Input: part model. Units: mm. Frame: model coordinates. Coordinates: 2 decimals unless noted, no trailing zeros. Write item = value, one per line. Start each with the question number.
from build123d import *

# Parameters (mm, degrees)
SHELL1_T                = -1.2
SKETCH5_W               = 1.35
SKETCH5_H               = 5.256968873
SKETCH5_H_2             = 1.35
SKETCH5_W_2             = 5.491330354
SKETCH5_W_3             = 5.273072972
SKETCH5_H_3             = 5.618351113
BOSS_EXTRUDE1_DEPTH     = 4
SKETCH6_R               = 2.5
BOSS_EXTRUDE2_DEPTH     = 10
CUT_EXTRUDE3_DEPTH      = 10
CUT_EXTRUDE3_DEPTH_BACK = 10
CUT_EXTRUDE4_DEPTH      = 0.5


with BuildPart() as part:
    # Loft1: read off the stored shape, not the designer's step
    # Loft1: loft between two sections, ruled curve by curve
    loft1_from = [
        Edge.make_line((-10, 0, 9.05), (-10, 0, -9.05)),
        Edge.make_line((-10, 0, -9.05), (10, 0, -9.05)),
        Edge.make_line((10, 0, 9.05), (-10, 0, 9.05)),
        Edge.make_line((10, 0, -9.05), (10, 0, 9.05)),
    ]
    loft1_to = [
        Edge.make_line((-7.5, 10, 6.318777005), (-7.5, 10, -7.681222995)),
        Edge.make_line((-7.5, 10, -7.681222995), (7.5, 10, -7.681222995)),
        Edge.make_line((7.5, 10, 6.318777005), (-7.5, 10, 6.318777005)),
        Edge.make_line((7.5, 10, -7.681222995), (7.5, 10, 6.318777005)),
    ]
    loft1 = Solid(Shell([*[Face.make_surface_from_curves(loft1_from[k], loft1_to[k]) for k in range(4)], Face(Wire(loft1_from)), Face(Wire(loft1_to))]))
    add(loft1)

    # Shell1
    shell1_openings = [part.faces().sort_by_distance(p)[0] for p in [
        (0, 0, 0),
    ]]
    offset(amount=SHELL1_T, openings=shell1_openings, kind=Kind.INTERSECTION)

    # Sketch5 → Boss-Extrude1 (add)
    with BuildSketch(Plane(origin=(0, 10, 0), x_dir=(1, 0, 0), z_dir=(0, 1, 0))):
        with Locations((0, -2.44038684)):
            Rectangle(SKETCH5_W, SKETCH5_H)
        with Locations((0, 0.863097596)):
            Rectangle(SKETCH5_W, SKETCH5_H_2)
        with Locations((3.420665177, 0.863097596)):
            Rectangle(SKETCH5_W_2, SKETCH5_H_2)
        with Locations((-3.311536486, 0.863097596)):
            Rectangle(SKETCH5_W_3, SKETCH5_H_2)
        with Locations((0, 4.347273152)):
            Rectangle(SKETCH5_W, SKETCH5_H_3)
    extrude(amount=-BOSS_EXTRUDE1_DEPTH)

    # Sketch6 → Boss-Extrude2 (add)
    with BuildSketch(Plane(origin=(0, 10, 0), x_dir=(1, 0, 0), z_dir=(0, 1, 0))):
        with Locations(Location((0, 0.829201721, 0), (0, 0, 270))):
            Circle(SKETCH6_R)
        Polygon((-0.675, 2.913097596), (-0.675, 1.538097596), (-2.05, 1.538097596), (-2.05, 0.188097596), (-0.675, 0.188097596), (-0.675, -1.186902404), (0.675, -1.186902404), (0.675, 0.188097596), (2.05, 0.188097596), (2.05, 1.538097596), (0.675, 1.538097596), (0.675, 2.913097596), align=None, mode=Mode.SUBTRACT)
    extrude(amount=-BOSS_EXTRUDE2_DEPTH)

    # Sketch4 → Cut-Extrude3 (cut, two sides: drawn at the far end of the back side and taken through both)
    with BuildSketch(Plane.XY.offset(-CUT_EXTRUDE3_DEPTH_BACK)):
        with BuildLine():
            Line((-7.5, 10), (7.5, 10))
            add(Edge.make_bspline(
                [(-7.5, 10), (-3.102300298, 9.460265696), (2.493912061, 9.41154423), (7.5, 10)],
                knots=[0, 0, 0, 0, 1, 1, 1, 1], degree=3))
        make_face()
    extrude(amount=CUT_EXTRUDE3_DEPTH + CUT_EXTRUDE3_DEPTH_BACK, mode=Mode.SUBTRACT)

    # Sketch7 → Cut-Extrude4 (cut)
    with BuildSketch(Plane(origin=(0, 10, 0), x_dir=(1, 0, 0), z_dir=(0, 1, 0))):
        with BuildLine():
            Line((-4.780864366, 5.922144036), (-3.519005391, 5.922144036))
            Line((-3.519005391, 5.922144036), (-3.519005391, 5.718618395))
            Line((-3.519005391, 5.718618395), (-3.637940688, 5.718618395))
            add(Edge.make_bspline(
                [(-3.637940688, 5.718618395), (-3.655135293, 5.718298675), (-3.686433195, 5.717716715), (-3.729006145, 5.712612802), (-3.763096016, 5.705393375), (-3.78881293, 5.692977812), (-3.8070942, 5.676915533), (-3.819447693, 5.657684085), (-3.827587368, 5.635286205), (-3.828346031, 5.619053057), (-3.828745976, 5.610495398)],
                knots=[0, 0, 0, 0, 1.655695587, 3.013724266, 4.12842979, 4.996263288, 5.734172721, 6.442363129, 7.178857587, 8, 8, 8, 8], degree=3))
            add(Edge.make_bspline(
                [(-3.828745976, 5.610495398), (-3.827935202, 5.596638054), (-3.8261785, 5.566613383), (-3.81792552, 5.537672623), (-3.813481553, 5.522088947)],
                knots=[0, 0, 0, 0, 0.92306383, 2, 2, 2, 2], degree=3))
            Line((-3.813481553, 5.522088947), (-3.132306673, 3.635660662))
            Line((-3.132306673, 3.635660662), (-2.586603548, 5.238425085))
            Line((-2.586603548, 5.238425085), (-2.691546457, 5.556433899))
            add(Edge.make_bspline(
                [(-2.691546457, 5.556433899), (-2.696705028, 5.569949091), (-2.7064075, 5.595369072), (-2.725520717, 5.629084688), (-2.747885349, 5.656076509), (-2.765681383, 5.669109501), (-2.774228749, 5.675369196)],
                knots=[0, 0, 0, 0, 1.175505941, 2.210944564, 3.140723652, 4, 4, 4, 4], degree=3))
            add(Edge.make_bspline(
                [(-2.774228749, 5.675369196), (-2.786526434, 5.682223978), (-2.812224647, 5.696548271), (-2.856749443, 5.708822147), (-2.906166524, 5.717600207), (-2.941028957, 5.718268145), (-2.959309879, 5.718618395)],
                knots=[0, 0, 0, 0, 0.875237679, 1.828965724, 2.861568027, 4, 4, 4, 4], degree=3))
            Line((-2.959309879, 5.718618395), (-3.111954109, 5.718618395))
            Line((-3.111954109, 5.718618395), (-3.111954109, 5.922144036))
            Line((-3.111954109, 5.922144036), (-1.605864366, 5.922144036))
            Line((-1.605864366, 5.922144036), (-1.605864366, 5.718618395))
            Line((-1.605864366, 5.718618395), (-1.747696297, 5.718618395))
            add(Edge.make_bspline(
                [(-1.747696297, 5.718618395), (-1.771456323, 5.718378199), (-1.814841431, 5.717939609), (-1.873911631, 5.711930572), (-1.920702063, 5.701790817), (-1.956628554, 5.687304501), (-1.982034107, 5.667479747), (-1.999396203, 5.643840507), (-2.011010812, 5.616593715), (-2.011847895, 5.596625547), (-2.01227963, 5.586326728)],
                knots=[0, 0, 0, 0, 1.714148818, 3.129985267, 4.276727023, 5.160657128, 5.901376261, 6.568437672, 7.261654719, 8, 8, 8, 8], degree=3))
            add(Edge.make_bspline(
                [(-2.01227963, 5.586326728), (-2.011825699, 5.576716145), (-2.010872101, 5.556526669), (-2.004700913, 5.537268169), (-2.001467331, 5.527177089)],
                knots=[0, 0, 0, 0, 0.952038799, 2, 2, 2, 2], degree=3))
            Line((-2.001467331, 5.527177089), (-1.381986161, 3.635660662))
            Line((-1.381986161, 3.635660662), (-0.8458233, 5.297574725))
            add(Edge.make_bspline(
                [(-0.8458233, 5.297574725), (-0.838138315, 5.322184666), (-0.82318736, 5.370062717), (-0.820871874, 5.420152039), (-0.819746577, 5.444494797)],
                knots=[0, 0, 0, 0, 1.028026033, 2, 2, 2, 2], degree=3))
            add(Edge.make_bspline(
                [(-0.819746577, 5.444494797), (-0.820535966, 5.465347045), (-0.822026939, 5.50473212), (-0.834869187, 5.560235902), (-0.856422532, 5.608480656), (-0.887535554, 5.648134893), (-0.924858201, 5.68006508), (-0.968418499, 5.702501412), (-1.017345761, 5.71638575), (-1.051795947, 5.717854835), (-1.069701505, 5.718618395)],
                knots=[0, 0, 0, 0, 1.192510613, 2.252376767, 3.240823701, 4.19251923, 5.11409438, 6.031584123, 6.976911646, 8, 8, 8, 8], degree=3))
            Line((-1.069701505, 5.718618395), (-1.158107956, 5.718618395))
            Line((-1.158107956, 5.718618395), (-1.158107956, 5.922144036))
            Line((-1.158107956, 5.922144036), (-0.14047975, 5.922144036))
            Line((-0.14047975, 5.922144036), (-0.14047975, 5.718618395))
            add(Edge.make_bspline(
                [(-0.14047975, 5.718618395), (-0.17000843, 5.716943894), (-0.226076597, 5.713764403), (-0.305801986, 5.6989593), (-0.375631822, 5.673331733), (-0.436896235, 5.639267674), (-0.489536795, 5.595758006), (-0.533856822, 5.542629255), (-0.570593733, 5.479973415), (-0.588077676, 5.433567924), (-0.597140407, 5.409513827)],
                knots=[0, 0, 0, 0, 1.193473395, 2.266131314, 3.259941233, 4.183600984, 5.083354208, 6.00064656, 6.963643304, 8, 8, 8, 8], degree=3))
            Line((-0.597140407, 5.409513827), (-1.482476946, 2.665733779))
            Line((-1.482476946, 2.665733779), (-1.745788244, 2.665733779))
            Line((-1.745788244, 2.665733779), (-2.482296657, 4.917236183))
            Line((-2.482296657, 4.917236183), (-3.249333917, 2.665733779))
            Line((-3.249333917, 2.665733779), (-3.471940087, 2.665733779))
            Line((-3.471940087, 2.665733779), (-4.515008997, 5.556433899))
            add(Edge.make_bspline(
                [(-4.515008997, 5.556433899), (-4.51937065, 5.570536793), (-4.527519997, 5.596886752), (-4.543498142, 5.632455097), (-4.561438603, 5.66146931), (-4.582786932, 5.683346509), (-4.606156722, 5.69999819), (-4.632897529, 5.710346771), (-4.662128217, 5.718097638), (-4.682858161, 5.718439241), (-4.693729951, 5.718618395)],
                knots=[0, 0, 0, 0, 1.34073981, 2.505048815, 3.536764225, 4.422637444, 5.267304403, 6.122676221, 7.015440249, 8, 8, 8, 8], degree=3))
            Line((-4.693729951, 5.718618395), (-4.780864366, 5.718618395))
            Line((-4.780864366, 5.718618395), (-4.780864366, 5.922144036))
        make_face()
    extrude(amount=-CUT_EXTRUDE4_DEPTH, mode=Mode.SUBTRACT)


solid = part.part
Item 1: Ray query, line 1 (Z direction, x = 1.5, y = 7.5); line 2 (X direction, y = 8.75, z = 1.75) (1 decimal); line 3 (X direction, y = 8.5, z = 1) (3 decimals). Return the intervals inside material, ascending.
Item 2: Pin query (flat end, axial travel): pin 1 (0.7 mm diameter, centred on y = 4, z = -0.5, fed in from -X); pin 2 (2 mm diameter, centred on x = -1, y = 6.5, fed in from +Z); pin 3 (2 mm diameter, centred on x = 2, y = 7.5, fed in from -Z). Return the tip coordinate at first contact, or that it passes through.
Item 3: Pull-direction query (X, two-part tool) for faces 1 (the cylindrical face through (0.751, 4.462, 1.555)), 2 (the flat face through (0, 0, 8)); classes: pulls with the +X half, pulls with the -X half, needs draft (parallel to the pull), parting line crosses it, or undercut.
Item 4: Cut plane A-A on y = 1.5. State how many separate pieces and enclosed holes the cut face has, plus the area to 3 significant figures.
Recorded:
q1.line_1 = -8.02 to -6.81, -2.83 to 1.17, 5.76 to 7
q1.line_2 = -7.8 to -6.6, -0.7 to 0.7, 6.6 to 7.8
q1.line_3 = -7.875 to -6.638, -1.704 to 1.704, 6.638 to 7.875
q2.pin_1 = -9.09
q2.pin_2 = 7.55
q2.pin_3 = -8.16
q3.face_1 = undercut
q3.face_2 = needs draft
q4.separate_pieces = 2
q4.enclosed_holes = 2
q4.area = 94.8 mm²
